Job drawing, mm, ordinate dimensions from the low corner. One solid piece. Give positions to 0.01 mm unless a question says otherwise; leave off trailing zeros. Order: outer loops, then holes, each group sorted by start corner. A loop starts at its lowest first (then second) coordinate and runs counter-clockwise, first axis right, second up.
Item 1: Band-saw the part on A-A on x = 167.64. Give the cut face in (y, z), plus the area to 3 significant figures.
Item 2: Band-saw the part on B-B on z = 7.25. Give the cut face in (x, y).
Item 3: Flat gauge pin, fed straight in: P1, Ø8, axis at x = 274, y = 91, coming from the +Z side. Where does the tip first touch, or does it go through?
Item 4: Wall check: L1, parallel to Y at x = 167.64, z = 3.5; L2, parallel to Y at x = 58.5, z = 3.75. Give the ranges that are in metal, low to high.
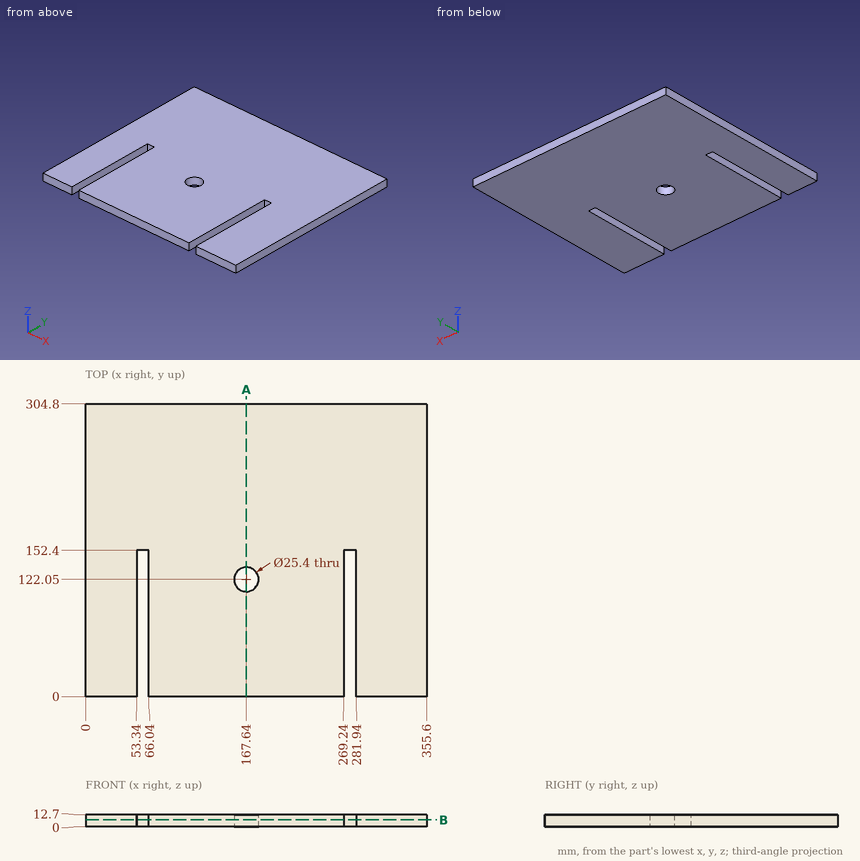
The answers:
1. outline: (0, 0) - (109.35, 0) - (109.35, 12.7) - (0, 12.7) - close; (134.75, 0) - (304.8, 0) - (304.8, 12.7) - (134.75, 12.7) - close
1. area: 3,550 mm2
2. outline: (0, 0) - (53.34, 0) - (53.34, 152.4) - (66.04, 152.4) - (66.04, 0) - (269.24, 0) - (269.24, 152.4) - (281.94, 152.4) - (281.94, 0) - (355.6, 0) - (355.6, 304.8) - (0, 304.8) - close; hole circle Ø25.4 at (167.64, 122.05)
3. P1: passes through
4. L1: y = 0 to 109.35, 134.75 to 304.8
4. L2: y = 152.4 to 304.8
